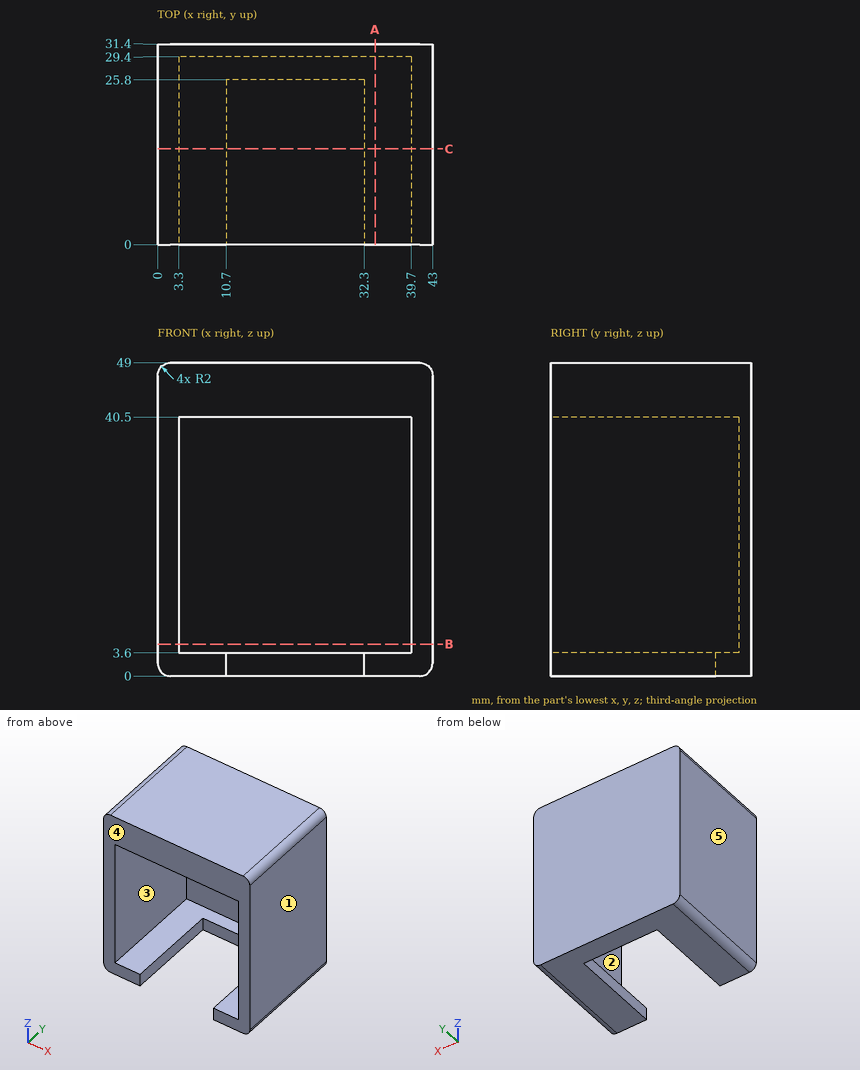
Part print with two shaded views. Sizes in mm from the minimum x, y, z corner. A direction names the side the tool comes from. Round coordinates to 2 decimals unless told otherwise and drop trailing zeros. Loops run counter-clockwise (first coordinate to the right, second up) from the corner with the lowest first, then second, coordinate; pieces in that order, holes last.
1. Slice it at A-A (x = 34). Give the cut face in (y, z).
Solutions:
outline: (0, 0) - (31.4, 0) - (31.4, 49) - (0, 49) - (0, 40.5) - (29.4, 40.5) - (29.4, 3.6) - (0, 3.6) - close
2. Slice it at B-B (z = 5). Give the cut face in (x, y), and give its area (3 significant figures).
Solutions:
outline: (0, 0) - (3.3, 0) - (3.3, 29.4) - (39.7, 29.4) - (39.7, 0) - (43, 0) - (43, 31.4) - (0, 31.4) - close
area: 280 mm2
3. Flat gauge pins, fed straight in: pin 1 (3 mm diameter, centred on x = 23.5, z = 1.5, fed in from -Y); pin 2 (11 mm diameter, centred on x = 21, z = 20, fed in from -Y). Where does each tip first touch, or does it go through?
Solutions:
pin 1: stops at y = 25.8
pin 2: stops at y = 29.4
4. Drill centre lines: line 1 along X through (y, z) = (14.5, 26); line 2 along Z through (x, y) = (6.5, 13); line 3 along Y through (x, z) = (10.5, 30). Where is each one in solid material? Low to high.
Solutions:
line 1: x = 0 to 3.3, 39.7 to 43
line 2: z = 0 to 3.6, 40.5 to 49
line 3: y = 29.4 to 31.4
5. 3-axis set-ups, long thin cutter, end or side, ignore diameter. For the marked faces 1 and 2: which of +Z, -Z, +X, -X, +Y, -Y reach the whole face in a straight line?
Solutions:
face 1: +Z, -Z, +X, +Y, -Y
face 2: -Y
6. Two-plate mould, pull along X, no slides. Class the marked faces 3, 4 and 5: pulls with the +X half, pulls with the -X half, needs draft (parallel to the pull), parting line crosses it, or undercut.
Solutions:
face 3: undercut
face 4: needs draft
face 5: pulls with the -X half
7. Slice it at C-C (y = 15). Give the cut face in (x, z).
Solutions:
outline: (0, 2) arc R2 ccw to (2, 0) - (10.7, 0) - (10.7, 3.6) - (3.3, 3.6) - (3.3, 40.5) - (39.7, 40.5) - (39.7, 3.6) - (32.3, 3.6) - (32.3, 0) - (41, 0) arc R2 ccw to (43, 2) - (43, 47) arc R2 ccw to (41, 49) - (2, 49) arc R2 ccw to (0, 47) - close
